from build123d import *

# Parameters (mm, degrees)
F2_R = 3


# Not quite as in the source:
# - a feature names something its author has since deleted; it is built from what else it names


with BuildPart() as f1:
    # F0 (on Front) → F1 (revolve)
    with BuildSketch(Plane.XZ):
        Polygon((-30, 0.1), (-30, 3), (-28.8, 4.2), (-28.8, 4.9), (-30, 6.1), (-30, 7.6), (-27.2, 7.6), (-27.2, 9.1), (-31.2, 9.1), (-31.7, 8.2339745962), (-31.7, 6.1), (-31.2, 5.6), (-31.2, 3.6), (-31.7, 3.1), (-31.7, 0.1), align=None)
    revolve(axis=Axis((0, 0, 8.878365159), (0, 0, 1)))

    # F2
    f2_edges = [f1.edges().sort_by_distance(p)[0] for p in [
        (31.7, 0, 8.233975),
    ]]
    fillet(f2_edges, radius=F2_R)


solid = f1.part
The listing builds one solid part. Answer for the finished solid, in the listing's coordinates (mm). A direction names the side the tool comes from. Coordinates: 2 decimals unless noted, no trailing zeros. Answer as CSV lines item,"result".
1. Determine the mould class of faces 1 (the conical face through (21, -20, 4)), 2 (the cylindrical face through (29.97, -1.32, 6.86)), 3 (the cylindrical face through (-30.236, -9.522, 1.579)) for opening direction Z: +Z half, -Z half, draft (parallel to the pull), parting line (faces both ways), or undercut.
Computed values:
face 1,"-Z half"
face 2,"undercut"
face 3,"draft"
2. Straight lines are drawn through the part: line 1 (X direction, y = 0, z = 1.1); line 2 (X direction, y = 0, z = 4.4). For each, find the intervals that lie inside material, in ascending order. Write a range as [from, to].
Computed values:
line 1,"x = [-31.7, -30], [30, 31.7]"
line 2,"x = [-31.2, -28.8], [28.8, 31.2]"
3. A tool of negligible diameter and unlimited length cuts with its end or side. For faces 4 (the cylindrical face through (-27.47, -8.65, 4.55)), 5 (the flat face through (-7, 27, 7.6)), 6 (the flat face through (-9, -26, 9.1)), from which of +Z, -Z, +X, -X, +Y, -Y can it reach the whole face along a straight path? Write none if from no direction.
Computed values:
face 4,"-Z"
face 5,"none"
face 6,"+Z, +X, -X, +Y, -Y"
4. Given P1, Ø1, axis at y = 3.5, z = 1, coming from the +X side; P2, Ø1.5, axis at x = -18.5, z = 1.5, coming from the +Y side; P3, Ø3, axis at x = -7.5, z = 6, coming from the +Y side; P4, Ø3, axis at x = -19.5, y = -17, coming from the +Z side, each flat-ended and moving along its own axis, determine where each tip first touches the part or whether it passes through.
Computed values:
P1,"stops at x = 31.56"
P2,"stops at y = 26.26"
P3,"stops at y = 31.13"
P4,"stops at z = 9.1"
